Check sheet for the modelled part. Datum: model origin and axes. Units: mm. A direction names the side the tool comes from. Round coordinates to 2 decimals unless told otherwise and drop trailing zeros. Loops run counter-clockwise (first coordinate to the right, second up) from the corner with the lowest first, then second, coordinate; pieces in that order, holes last. Notation, with made-up numbers: M 3,85.25 L 61,85.25 A19 cw 61,103.25 Z; hole C -12.75,71.25 d10. An arc over 180 degrees is marked long. One line per question, with ' | ' between items. Start each with the question number.
(1) Section check A-A (z = -2). Record the boundary of the cut face in (x, y).
(2) Draft check along X on faces 1 (the face through (2, 36, -5)), 2 (the face through (-53.795, 30.538, 1.972)), 3 (the face through (-58.1, 4, 4)). Enter one of: +X half, -X half, draft (parallel to the pull), parting line (faces both ways), or undercut.
(3) Go/stop test with flat-tipped pins: P1, Ø21, axis at x = -33, y = 16.5, coming from the +Z side; P2, Ø3.5, axis at x = -53.6, y = -21.95, coming from the -Z side; P3, Ø1, axis at x = -2.5, z = 5, coming from the -Y side; P4, Ø4, axis at x = 23, z = 14, coming from the +Y side. Record where each tip stops, or that it passes through.
(4) Section check D-D (z = 12.75). Record the boundary of the cut face in (x, y), and give its area (3 significant figures).
(5) Tool access check on faces 4 (the face through (41, 33.55, 4)), 5 (the face through (54.403, -21.818, 6.465)), 6 (the face through (-3.45, 36, 9)), 7 (the face through (41, -26.45, 4)). Record the directions out of +Z, -Z, +X, -X, +Y, -Y that give a thin tool (end or side, any length) a straight path to the whole face; none if there is none.
(6) Thickness scan on probe 1 along Y at (x, z) = (-19, 6); probe 2 along Z at (x, y) = (56, 0); probe 3 along X at (y, z) = (-22.5, 3.25). Record the ranges inside material, lowest first. Write a range as [from, to].
(7) Section check C-C (x = 13.5). Record the boundary of the cut face in (y, z), and give its area (3 significant figures).
(8) Section check B-B (y = 22.5). Record the boundary of the cut face in (x, z).
```python
from build123d import *
from build123d.topology import SkipClean

# Parameters (mm, degrees)
SKETCH1_R               = 35
SKETCH1_R_2             = 33.5
BOSS_EXTRUDE1_DEPTH     = 20
SKETCH1_5_R             = 3
SKETCH1_5_R_2           = 1.5
BOSS_EXTRUDE3_DEPTH     = 4
BOSS_EXTRUDE3_2_DEPTH   = 4
BOSS_EXTRUDE3_3_DEPTH   = 4
BOSS_EXTRUDE3_4_DEPTH   = 4
SKETCH1_6_R             = 3
BOSS_EXTRUDE4_DEPTH     = 9
CUT_EXTRUDE2_DEPTH      = 22
CUT_EXTRUDE2_DEPTH_BACK = 76
SKETCH3_W               = 10.7
SKETCH3_H               = 12.2
SKETCH5_R               = 35
SKETCH5_R_2             = 31.5
BOSS_EXTRUDE9_DEPTH     = 20
BOSS_EXTRUDE11_START    = 5
BOSS_EXTRUDE11_DEPTH    = 5
CUT_EXTRUDE3_DEPTH      = 22
CUT_EXTRUDE3_DEPTH_BACK = 92
SKETCH3_2_W             = 10.7
SKETCH3_2_H             = 12.2


with BuildPart() as part:
    # Sketch1 → Boss-Extrude1 (new body)
    with BuildSketch(Plane.XY):
        with Locations((1.900049518, 3.550317981)):
            Circle(SKETCH1_R)
        with Locations((1.900049518, 3.550317981)):
            Circle(SKETCH1_R_2, mode=Mode.SUBTRACT)
    extrude(amount=BOSS_EXTRUDE1_DEPTH)



with BuildPart() as body_2:
    # Sketch1_5 → Boss-Extrude3 (new body)
    with BuildSketch(Plane.XY):
        with Locations((57.400049518, 29.050317981)):
            Circle(SKETCH1_5_R)
        with Locations((57.400049518, 29.050317981)):
            Circle(SKETCH1_5_R_2, mode=Mode.SUBTRACT)
    extrude(amount=BOSS_EXTRUDE3_DEPTH)


with BuildPart() as body_3:
    # Sketch1_5 → Boss-Extrude3 2 (new body)
    with BuildSketch(Plane.XY):
        with Locations((-53.599950482, 29.050317981)):
            Circle(SKETCH1_5_R)
        with Locations((-53.599950482, 29.050317981)):
            Circle(SKETCH1_5_R_2, mode=Mode.SUBTRACT)
    extrude(amount=BOSS_EXTRUDE3_2_DEPTH)


with BuildPart() as body_4:
    # Sketch1_5 → Boss-Extrude3 3 (new body)
    with BuildSketch(Plane.XY):
        with Locations((-53.599950482, -21.949682019)):
            Circle(SKETCH1_5_R)
        with Locations((-53.599950482, -21.949682019)):
            Circle(SKETCH1_5_R_2, mode=Mode.SUBTRACT)
    extrude(amount=BOSS_EXTRUDE3_3_DEPTH)


with BuildPart() as body_5:
    # Sketch1_5 → Boss-Extrude3 4 (new body)
    with BuildSketch(Plane.XY):
        with Locations((57.400049518, -21.949682019)):
            Circle(SKETCH1_5_R)
        with Locations((57.400049518, -21.949682019)):
            Circle(SKETCH1_5_R_2, mode=Mode.SUBTRACT)
    extrude(amount=BOSS_EXTRUDE3_4_DEPTH)


with BuildPart() as part_1:
    add(part.part)

    add(body_2.part)  # Boss-Extrude4 merges body 2

    add(body_3.part)  # Boss-Extrude4 merges body 3

    add(body_4.part)  # Boss-Extrude4 merges body 4

    add(body_5.part)  # Boss-Extrude4 merges body 5
    # Sketch1_6 → Boss-Extrude4 (add)
    # profile 1 of 2: a face of its own
    with BuildSketch(Plane.XY):
        with BuildLine():
            Line((-16.12770686, 33.550317981), (-58.099950482, 33.550317981))
            Line((-58.099950482, 33.550317981), (-58.099950482, -26.449682019))
            Line((-58.099950482, -26.449682019), (-16.12770686, -26.449682019))
            ThreePointArc((-16.12770686, -26.449682019), (-33.099950482, 3.550317981), (-16.12770686, 33.550317981))
        make_face()
        with Locations((-53.599950482, -21.949682019)):
            Circle(SKETCH1_6_R, mode=Mode.SUBTRACT)
        with Locations((-53.599950482, 29.050317981)):
            Circle(SKETCH1_6_R, mode=Mode.SUBTRACT)
    # profile 2 of 2: a face of its own
    with BuildSketch(Plane.XY):
        with BuildLine():
            Line((61.900049518, 33.550317981), (19.927805895, 33.550317981))
            ThreePointArc((19.927805895, 33.550317981), (32.362907831, 20.784419739), (36.900049518, 3.550317981))
            ThreePointArc((36.900049518, 3.550317981), (32.362907831, -13.683783776), (19.927805895, -26.449682019))
            Line((19.927805895, -26.449682019), (61.900049518, -26.449682019))
            Line((61.900049518, -26.449682019), (61.900049518, 33.550317981))
        make_face()
        with Locations((57.400049518, -21.949682019)):
            Circle(SKETCH1_6_R, mode=Mode.SUBTRACT)
        with Locations((57.400049518, 29.050317981)):
            Circle(SKETCH1_6_R, mode=Mode.SUBTRACT)
    extrude(amount=BOSS_EXTRUDE4_DEPTH)

    # Sketch3 → Cut-Extrude2 (cut, two sides: drawn at the far end of the back side and taken through both)
    with BuildSketch(Plane(origin=(0, -26.449682019, 0), x_dir=(-1, 0, 0), z_dir=(0, -1, 0)).offset(-CUT_EXTRUDE2_DEPTH_BACK)):
        with Locations((-1.900049518, -8.9)):
            Rectangle(SKETCH3_W, SKETCH3_H)
    extrude(amount=CUT_EXTRUDE2_DEPTH + CUT_EXTRUDE2_DEPTH_BACK, mode=Mode.SUBTRACT)

    # Sketch5 → Boss-Extrude9 (add)
    with BuildSketch(Plane(origin=(0, 0, 0), x_dir=(-1, 0, 0), z_dir=(0, 0, -1))):
        with Locations(Location((-1.900049518, 3.550317981, 0), (0, 0, 58.997280866))):
            Circle(SKETCH5_R)
        with Locations((-1.900049518, 3.550317981)):
            Circle(SKETCH5_R_2, mode=Mode.SUBTRACT)
    extrude(amount=-BOSS_EXTRUDE9_DEPTH)

    # Sketch5_11 → Boss-Extrude11 (add)
    with SkipClean():  # the faces are left unmerged after this step: merging them gives an invalid solid
        with BuildSketch(Plane(origin=(0, 0, 0), x_dir=(-1, 0, 0), z_dir=(0, 0, -1)).offset(BOSS_EXTRUDE11_START)):
            with BuildLine():
                ThreePointArc((16.12770686, 33.550317981), (-1.900049518, 38.550317981), (-19.927805895, 33.550317981))
                Line((-19.927805895, 33.550317981), (-10.647592465, 33.811357163))
                ThreePointArc((-10.647592465, 33.811357163), (-1.900049518, 35.050317981), (6.84749343, 33.811357163))
                Line((6.84749343, 33.811357163), (16.12770686, 33.550317981))
            make_face()
            with BuildLine():
                ThreePointArc((6.84749343, 33.811357163), (-1.900049518, 35.050317981), (-10.647592465, 33.811357163))
                Line((-10.647592465, 33.811357163), (6.84749343, 33.811357163))
            make_face()
            with BuildLine():
                ThreePointArc((-10.647592465, -26.710721201), (-1.900049518, -27.949682019), (6.84749343, -26.710721201))
                Line((6.84749343, -26.710721201), (-10.647592465, -26.710721201))
            make_face()
            with BuildLine():
                ThreePointArc((-19.927805895, -26.449682019), (-1.900049518, -31.449682019), (16.12770686, -26.449682019))
                Line((16.12770686, -26.449682019), (6.84749343, -26.710721201))
                ThreePointArc((6.84749343, -26.710721201), (-1.900049518, -27.949682019), (-10.647592465, -26.710721201))
                Line((-10.647592465, -26.710721201), (-19.927805895, -26.449682019))
            make_face()
        extrude(amount=-BOSS_EXTRUDE11_DEPTH)

    # Sketch3_2 → Cut-Extrude3 (cut, two sides: drawn at the far end of the back side and taken through both)
    with SkipClean():  # the faces are left unmerged after this step: merging them gives an invalid solid
        with BuildSketch(Plane(origin=(0, -26.449682019, 0), x_dir=(-1, 0, 0), z_dir=(0, -1, 0)).offset(-CUT_EXTRUDE3_DEPTH_BACK)):
            with Locations((-1.900049518, -8.9)):
                Rectangle(SKETCH3_2_W, SKETCH3_2_H)
        extrude(amount=CUT_EXTRUDE3_DEPTH + CUT_EXTRUDE3_DEPTH_BACK, mode=Mode.SUBTRACT)


solid = part_1.part
```
The answers:
1) outline: M -16.13,-26.45 A35 ccw 19.93,-26.45 L 10.65,-26.71 L -6.85,-26.71 Z; M -16.13,33.55 L -6.85,33.81 L 10.65,33.81 L 19.93,33.55 A35 ccw Z
2) face 1: draft | face 2: undercut | face 3: -X half
3) P1: z = 20 | P2: z = 0 | P3: through | P4: y = 32.88
4) outline: M -3.45,-31.04 L -3.45,-27.49 A31.5 cw -3.45,34.59 L -3.45,38.14 A35 ccw Z; M 7.25,-31.04 A35 ccw 7.25,38.14 L 7.25,34.59 A31.5 cw 7.25,-27.49 Z | area: 656 mm²
5) face 4: +Z, -Z, +X, +Y | face 5: +Z | face 6: +Y, -Y | face 7: +Z, -Z, +X, -Y
6) probe 1: [-26.45, -20.02], [27.12, 33.55] | probe 2: [0, 9] | probe 3: [-58.1, -55], [-52.2, -15.81], [19.61, 56], [58.8, 61.9]
7) outline: M -29.47,-5 L -26.63,-5 L -26.63,0 L -25.74,0 L -25.74,20 L -29.47,20 Z; M 32.84,0 L 33.73,0 L 33.73,-5 L 36.57,-5 L 36.57,20 L 32.84,20 Z | area: 178 mm²
8) outline: M -58.1,0 L -23.26,0 L -23.26,20 L -27.53,20 L -27.53,9 L -58.1,9 Z; M 27.06,0 L 61.9,0 L 61.9,9 L 31.33,9 L 31.33,20 L 27.06,20 Z
